Work out the finished part from the listing and answer in its coordinate system (mm). A direction names the side the tool comes from. Give positions to 0.01 mm unless a question says otherwise; leave off trailing zeros. Loops run counter-clockwise (first coordinate to the right, second up) from the corner with the lowest first, then second, coordinate; pieces in that order, holes last. Notation, with made-up numbers: (-13, -37.75) - (29, -37.75) arc R5 cw to (29, -29.75) - close; hole circle Ø7 at (-32, -14.5). An arc over 180 degrees is marked (long way). One line per question, with ' | ' between items. Start each with the question number.
1. Find the intervals of material crossed by line 1 (Z direction, x = 0, y = 5); line 2 (Z direction, x = 2, y = 3.25); line 3 (Y direction, x = -13, z = 12), in increasing order.
2. Section C-C (x = 5) is taken. Determine the outline of the cut face in (y, z).
3. Section D-D (y = 1.25) is taken. Give the number of separate pieces and of enclosed holes in the cut face, plus the area to 3 significant figures.
4. Which of the six approach directions +Z, -Z, +X, -X, +Y, -Y give full straight-line access (tool end or side, diameter ignored) to faces 4 (the face through (-16, -1, -7.5)), 5 (the face through (3.1, 1, 23)), 6 (the face through (0, 2, 5.839)), 7 (the face through (16, -2, 7.5)), 8 (the face through (-16, -1, 7.5))?
5. Section A-A (y = -3) is taken. Determine the outline of the cut face in (x, z).
6. For a pull along X with two mould halves and no side action, classify faces 1 (the face through (0, 4, -14.036)), 2 (the face through (-14.7, 1, -22)), 3 (the face through (-3.1, 1, 23)) as released by +X, released by -X, zero draft, split by the parting line, or undercut.
7. Section B-B (x = 0) is taken. Determine the outline of the cut face in (y, z), plus the area to 3 significant figures.
8. Each of these flat-tipped pins is pushed along its axis until it touches: pin 1 (3 mm diameter, centred on x = 3, z = 2, fed in from -Y); pin 2 (3 mm diameter, centred on x = -2.5, z = 26, fed in from +Y); pin 3 (3.5 mm diameter, centred on x = -9.525, z = 24.875, fed in from -Y). Where does it stop, or does it pass through?
from build123d import *

# Parameters (mm, degrees)
SKETCH1_W               = 29.4
SKETCH1_H               = 73.9
SKETCH1_W_2             = 15.82
SKETCH1_H_2             = 7.1
SKETCH1_W_3             = 6.2
SKETCH1_H_3             = 4.8
BOSS_EXTRUDE1_DEPTH     = 2
SKETCH1_3_R             = 6.875
BOSS_EXTRUDE2_DEPTH     = 10
SHELL1_T                = -0.75
SKETCH1_4_W             = 19.75
SKETCH1_4_H             = 20.75
BOSS_EXTRUDE3_DEPTH     = 5.4
SKETCH2_W               = 19
SKETCH2_H               = 19
CUT_EXTRUDE1_DEPTH      = 4.4
CUT_EXTRUDE2_DEPTH      = 41.563437971
CUT_EXTRUDE2_DEPTH_BACK = 41.563437971
SKETCH5_W               = 15
SKETCH5_H               = 1
SKETCH5_W_2             = 7.5
SKETCH5_H_2             = 2
BOSS_EXTRUDE4_DEPTH     = 0.75
SKETCH6_W               = 15
SKETCH6_H               = 7.47
BOSS_EXTRUDE5_DEPTH     = 1
MIRROR1_START           = -7.5
MIRROR1_DEPTH           = 15


# Read off the part's stored shape, not the designer's step: Mirror1
with BuildPart() as part:
    # Sketch1 → Boss-Extrude1 (new body)
    with BuildSketch(Plane(origin=(0, 0, 0), x_dir=(1, 0, 0), z_dir=(0, 1, 0))):
        Rectangle(SKETCH1_W, SKETCH1_H)
        with Locations((0, -30.932)):
            Rectangle(SKETCH1_W_2, SKETCH1_H_2, mode=Mode.SUBTRACT)
        with Locations((0, -23.449)):
            Rectangle(SKETCH1_W_3, SKETCH1_H_3, mode=Mode.SUBTRACT)
        with BuildLine():
            Line((-9.875, 14.036), (9.875, 14.036))
            Line((9.875, 14.036), (9.875, -6.714))
            Line((9.875, -6.714), (2.239559108, -6.714))
            ThreePointArc((2.239559108, -6.714), (0, -20.089), (-2.239559108, -6.714))
            Line((-2.239559108, -6.714), (-9.875, -6.714))
            Line((-9.875, -6.714), (-9.875, 14.036))
        make_face(mode=Mode.SUBTRACT)
    extrude(amount=BOSS_EXTRUDE1_DEPTH)



with BuildPart() as body_2:
    # Sketch1<3> → Boss-Extrude2 (new body)
    with BuildSketch(Plane(origin=(0, 0, 0), x_dir=(1, 0, 0), z_dir=(0, 1, 0))):
        with Locations(Location((0, -13.214, 0), (0, 0, 270))):
            Circle(SKETCH1_3_R)
    extrude(amount=BOSS_EXTRUDE2_DEPTH)

    # Shell1
    shell1_openings = [body_2.faces().sort_by_distance(p)[0] for p in [
        (0, 0, 13.214),
    ]]
    offset(amount=SHELL1_T, openings=shell1_openings, kind=Kind.INTERSECTION)


with BuildPart() as part_1:
    add(part.part)

    add(body_2.part)  # Boss-Extrude3 merges body 2
    # Sketch1<4> → Boss-Extrude3 (add)
    with BuildSketch(Plane(origin=(0, 0, 0), x_dir=(1, 0, 0), z_dir=(0, 1, 0))):
        with Locations((0, 3.661)):
            Rectangle(SKETCH1_4_W, SKETCH1_4_H)
    extrude(amount=BOSS_EXTRUDE3_DEPTH)

    # Sketch2 → Cut-Extrude1 (cut)
    with BuildSketch(Plane.XZ):
        with Locations((0, -3.661)):
            Rectangle(SKETCH2_W, SKETCH2_H)
    extrude(amount=-CUT_EXTRUDE1_DEPTH, mode=Mode.SUBTRACT)

    # Sketch3 → Cut-Extrude2 (cut, two sides: drawn at the far end of the back side and taken through both)
    with BuildSketch(Plane(origin=(0, 2, 0), x_dir=(1, 0, 0), z_dir=(0, 1, 0)).offset(-CUT_EXTRUDE2_DEPTH_BACK)):
        with BuildLine():
            Line((-9.525, 30.775), (-9.525, 32.275))
            Line((-9.525, 32.275), (-8.025, 32.275))
            ThreePointArc((-8.025, 32.275), (-10.585660172, 33.335660172), (-9.525, 30.775))
        make_face()
        with BuildLine():
            Line((-8.025, 32.275), (-9.525, 32.275))
            Line((-9.525, 32.275), (-9.525, 30.775))
            ThreePointArc((-9.525, 30.775), (-8.464339828, 31.214339828), (-8.025, 32.275))
        make_face()
        with BuildLine():
            ThreePointArc((11.025, 32.275), (9.525, 33.775), (8.025, 32.275))
            Line((8.025, 32.275), (9.525, 32.275))
            Line((9.525, 32.275), (9.525, 30.775))
            ThreePointArc((9.525, 30.775), (10.585660172, 31.214339828), (11.025, 32.275))
        make_face()
        with BuildLine():
            Line((9.525, 32.275), (8.025, 32.275))
            ThreePointArc((8.025, 32.275), (8.464339828, 31.214339828), (9.525, 30.775))
            Line((9.525, 30.775), (9.525, 32.275))
        make_face()
        with BuildLine():
            ThreePointArc((11.025, -24.875), (10.585660172, -23.814339828), (9.525, -23.375))
            Line((9.525, -23.375), (9.525, -24.875))
            Line((9.525, -24.875), (8.025, -24.875))
            ThreePointArc((8.025, -24.875), (9.525, -26.375), (11.025, -24.875))
        make_face()
        with BuildLine():
            Line((9.525, -24.875), (9.525, -23.375))
            ThreePointArc((9.525, -23.375), (8.464339828, -23.814339828), (8.025, -24.875))
            Line((8.025, -24.875), (9.525, -24.875))
        make_face()
        with BuildLine():
            ThreePointArc((-8.025, -24.875), (-8.464339828, -23.814339828), (-9.525, -23.375))
            Line((-9.525, -23.375), (-9.525, -24.875))
            Line((-9.525, -24.875), (-8.025, -24.875))
        make_face()
        with BuildLine():
            Line((-9.525, -24.875), (-9.525, -23.375))
            ThreePointArc((-9.525, -23.375), (-10.585660172, -25.935660172), (-8.025, -24.875))
            Line((-8.025, -24.875), (-9.525, -24.875))
        make_face()
    extrude(amount=CUT_EXTRUDE2_DEPTH + CUT_EXTRUDE2_DEPTH_BACK, mode=Mode.SUBTRACT)

    # Sketch5 → Boss-Extrude4 (add)
    with BuildSketch(Plane(origin=(14.7, 0, 0), x_dir=(0, 0, -1), z_dir=(1, 0, 0))):
        with Locations((0, -4.97)):
            Rectangle(SKETCH5_W, SKETCH5_H)
        with Locations((-3.75, 1)):
            Rectangle(SKETCH5_W_2, SKETCH5_H_2)
        with Locations((3.75, 1)):
            Rectangle(SKETCH5_W_2, SKETCH5_H_2)
    extrude(amount=BOSS_EXTRUDE4_DEPTH)


with BuildPart() as boss_extrude4_piece_1:
    # of the separate pieces the step leaves, piece 1, a body of its own (boss_extrude4_pieces)
    add(part_1.part.solids().sort_by_distance((-14.7, 0, 36.95))[0])



with BuildPart() as boss_extrude4_piece_2:
    # of the separate pieces the step leaves, piece 2, a body of its own (boss_extrude4_pieces)
    add(part_1.part.solids().sort_by_distance((14.7, -4.47, -7.5))[0])


with BuildPart() as boss_extrude4_piece_1_1:
    add(boss_extrude4_piece_1.part)

    add(boss_extrude4_piece_2.part)  # Boss-Extrude5 merges Boss-Extrude4 piece 2
    # Sketch6 → Boss-Extrude5 (add)
    with BuildSketch(Plane(origin=(15.45, 0, 0), x_dir=(0, 0, -1), z_dir=(1, 0, 0))):
        with Locations((0, -1.735)):
            Rectangle(SKETCH6_W, SKETCH6_H)
    extrude(amount=BOSS_EXTRUDE5_DEPTH)

    # Mirror1 outline → Mirror1 (add)
    with BuildSketch(Plane.XY.offset(MIRROR1_START)):
        Polygon((-16.45, 2), (-16.45, -5.47), (-15.45, -5.47), (-15.45, 0), (-14.7, 0), (-14.7, 2), align=None)
    extrude(amount=MIRROR1_DEPTH)


solid = boss_extrude4_piece_1_1.part
Conclusion:
1) line 1: -14.04 to 7.09, 19.34 to 20.09 | line 2: -14.04 to -13.16, 5.84 to 7.42, 19 to 19.79 | line 3: 0 to 2
2) outline: (0, -36.95) - (2, -36.95) - (2, -14.04) - (5.4, -14.04) - (5.4, 6.71) - (2, 6.71) - (2, 8.5) - (10, 8.5) - (10, 17.93) - (2, 17.93) - (2, 27.38) - (0, 27.38) - (0, 16.75) - (9.25, 16.75) - (9.25, 9.68) - (0, 9.68) - (0, 5.84) - (4.4, 5.84) - (4.4, -13.16) - (0, -13.16) - close; (0, 34.48) - (2, 34.48) - (2, 36.95) - (0, 36.95) - close
3) separate pieces: 1 | enclosed holes: 8 | area: 1,580 mm²
4) face 4: -Z, -X, +Y, -Y | face 5: +Y, -Y | face 6: -Y | face 7: +Z, +X, +Y, -Y | face 8: +Z, -X, +Y, -Y
5) outline: (-16.45, -7.5) - (-15.45, -7.5) - (-15.45, 7.5) - (-16.45, 7.5) - close; (15.45, -7.5) - (16.45, -7.5) - (16.45, 7.5) - (15.45, 7.5) - close
6) face 1: zero draft | face 2: released by -X | face 3: undercut
7) outline: (0, -36.95) - (2, -36.95) - (2, -14.04) - (5.4, -14.04) - (5.4, 6.34) - (10, 6.34) - (10, 20.09) - (2, 20.09) - (2, 21.05) - (0, 21.05) - (0, 19.34) - (9.25, 19.34) - (9.25, 7.09) - (0, 7.09) - (0, 5.84) - (4.4, 5.84) - (4.4, -13.16) - (0, -13.16) - close; (0, 25.85) - (2, 25.85) - (2, 27.38) - (0, 27.38) - close; (0, 34.48) - (2, 34.48) - (2, 36.95) - (0, 36.95) - close | area: 106 mm²
8) pin 1: y = 4.4 | pin 2: y = 2 | pin 3: y = 0
